from build123d import *

# Parameters (mm, degrees)
WYTNIJ_WYCI_GNI_CIE1_DEPTH      = 33.908965344
WYTNIJ_WYCI_GNI_CIE1_DEPTH_BACK = 33.908965344
SZKIC2_R                        = 13
WYTNIJ_WYCI_GNI_CIE4_DEPTH      = 2
WYTNIJ_WYCI_GNI_CIE4_DEPTH_BACK = 2
SZKIC5_R                        = 19


with BuildPart() as part:
    # Szkic1 → Obr_t1 (revolve)
    with BuildSketch(Plane.XY, mode=Mode.PRIVATE) as obr_t1_sk:
        with BuildLine():
            ThreePointArc((0, 13), (-13, 0), (0, -13))
            Line((0, -13), (0, 13))
        make_face()
        with BuildLine():
            Line((0, 13), (0, -13))
            ThreePointArc((0, -13), (9.192388155, -9.192388155), (13, 0))
            ThreePointArc((13, 0), (9.192388155, 9.192388155), (0, 13))
        make_face()
        with BuildLine():
            Line((0, -13), (0, -19))
            ThreePointArc((0, -19), (19, 0), (0, 19))
            Line((0, 19), (0, 13))
            ThreePointArc((0, 13), (9.192388155, 9.192388155), (13, 0))
            ThreePointArc((13, 0), (9.192388155, -9.192388155), (0, -13))
        make_face()
    revolve(obr_t1_sk.sketch.rotate(Axis((0, -27.54752711, 0), (0, 1, 0)), 180), axis=Axis((0, -27.54752711, 0), (0, 1, 0)))

    # Szkic2 → Wytnij-wyci_gni_cie1 (cut, two sides: drawn at the far end of the back side and taken through both)
    with BuildSketch(Plane.XY.offset(-WYTNIJ_WYCI_GNI_CIE1_DEPTH_BACK)):
        with Locations(Location((0, 0, 0), (0, 0, 180))):
            Circle(SZKIC2_R)
    extrude(amount=WYTNIJ_WYCI_GNI_CIE1_DEPTH + WYTNIJ_WYCI_GNI_CIE1_DEPTH_BACK, mode=Mode.SUBTRACT)

    # Szkic5 → Wytnij-wyci_gni_cie4 (cut, two sides: drawn at the far end of the back side and taken through both)
    with BuildSketch(Plane(origin=(0, 0, 0), x_dir=(0, 0, -1), z_dir=(1, 0, 0)).offset(-WYTNIJ_WYCI_GNI_CIE4_DEPTH_BACK)):
        with Locations((0, 34)):
            Circle(SZKIC5_R)
    extrude(amount=WYTNIJ_WYCI_GNI_CIE4_DEPTH + WYTNIJ_WYCI_GNI_CIE4_DEPTH_BACK, mode=Mode.SUBTRACT)


solid = part.part
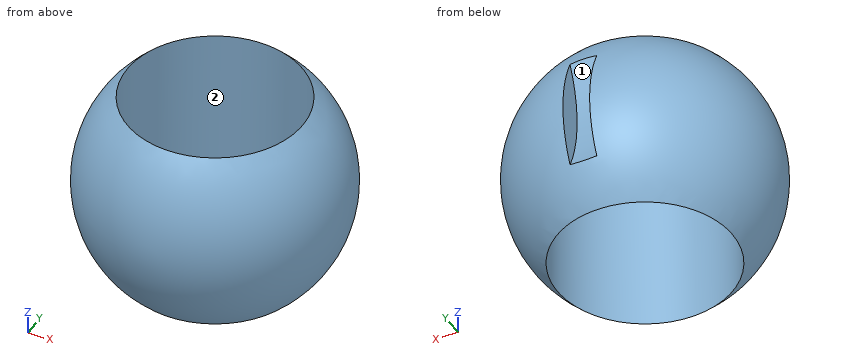
The model under review builds one solid part; all positions refer to its coordinate system, in mm. Face numbers are marked on the shaded views. Give positions to 0.01 mm unless a question says otherwise; leave off trailing zeros. Loops run counter-clockwise (first coordinate to the right, second up) from the corner with the lowest first, then second, coordinate; pieces in that order, holes last. Notation, with made-up numbers: (52, 51.5) -> (108, 51.5) arc R20 ccw to (108, 67.5) -> close; hole circle Ø5 at (5.25, 47). An arc over 180 degrees is marked (long way). Write each question's results on one line, items separated by ' | '.
1) Take a section at A-A, the plane x = 0. Give the boundary of the cut face in (y, z), plus the area to 3 significant figures.
Conclusion:
outline: (-13, -13.86) -> (-13, 13.86) arc R19 ccw to start; (13, -13.86) arc R19 ccw to (17, -8.49) arc R19 cw to (17, 8.49) arc R19 ccw to (13, 13.86) -> close | area: 184 mm^2
2) Take a section at D-D, the plane x = -11.5. Give the boundary of the cut face in (y, z), plus the area to 3 significant figures.
Conclusion:
outline: (-6.06, -13.86) -> (-6.06, 13.86) arc R15.12 ccw to start; (6.06, -13.86) arc R15.12 ccw to (6.06, 13.86) -> close | area: 362 mm^2
3) Insertion check: pin 1 Ø1 at (x, z) = (-13, -7) entering from +Y; pin 2 Ø1 at (x, z) = (10, 2) entering from +Y; pin 3 Ø1 at (x, y) = (3, 15) entering from +Z. Each pin has a flat end and moves straight along its axis. Give the tip position at first contact, or say it passes through.
Conclusion:
pin 1: stops at y = 12.55 | pin 2: stops at y = 16.34 | pin 3: stops at z = 11.92
4) For line 1 along X through (y, z) = (16, -5.5); line 2 along Y through (x, z) = (0, -7.25); line 3 along Y through (x, z) = (-8, 4.25), list the stretches that pass through material, from the lowest coordinate up. Write a range as from..to.
Conclusion:
line 1: x = -8.65..-2, 2..8.65 | line 2: y = -17.56..-13, 13..16.44 | line 3: y = -16.7..-10.25, 10.25..16.7
5) Take a section at B-B, the plane y = 0. Give the boundary of the cut face in (x, z).
Conclusion:
outline: (-13, -13.86) -> (-13, 13.86) arc R19 ccw to start; (13, -13.86) arc R19 ccw to (13, 13.86) -> close
6) Draft analysis for pull direction X (two halves, no side actions). For the marked faces 1 and 2, state which applies: pulls with the +X half, pulls with the -X half, needs draft (parallel to the pull), parting line crosses it, or undercut.
Conclusion:
face 1: undercut | face 2: undercut
7) Take a section at C-C, the plane z = 2.5. Give the boundary of the cut face in (x, y).
Conclusion:
outline: (-2, 15.17) -> (-2, 18.73) arc R18.83 ccw (long way) to (2, 18.73) -> (2, 15.17) -> close; hole circle Ø26 at (0, 0)
